Design review of the part shown in the three views and the two pictorial views. Dimensions are in mm from the part's minimum x, y and z. Give positions to 0.01 mm unless a question says otherwise; leave off trailing zeros. Loops run counter-clockwise (first coordinate to the right, second up) from the corner with the lowest first, then second, coordinate; pieces in that order, holes last. Notation, with made-up numbers: (31.25, 44) - (88.25, 44) arc R34 cw to (88.25, 76) - close; hole circle Ø7 at (-12, 36.25). An arc over 180 degrees is marked (long way). Answer in a Markdown table with one row per item.
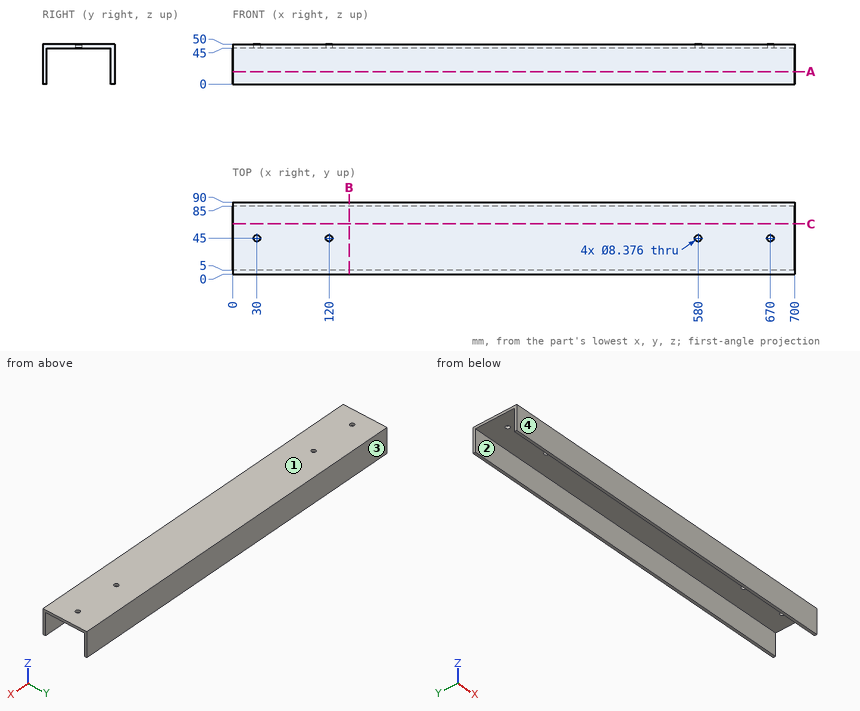
1. Wall thickness on line 1 (X direction, y = 45, z = 48.3); line 2 (Y direction, x = 563.5, z = 15.5); line 3 (Z direction, x = 207, y = 60.5): over which ranges is each line inside the solid? List them lowest first. Write a range as [from, to].
Values:
| item | result |
|---|---|
| line 1 | x = [0, 25.81], [34.19, 115.81], [124.19, 575.81], [584.19, 665.81], [674.19, 700] |
| line 2 | y = [0, 5], [85, 90] |
| line 3 | z = [45, 50] |
2. Clearance check with flat-ended pins moving along their axes: pin 1 (9.5 mm diameter, centred on x = 30, y = 45, fed in from +Z); pin 2 (1.5 mm diameter, centred on x = 471.5, y = 80.5, fed in from -Z). State where each tip first meets the part, or that it passes through.
Values:
| item | result |
|---|---|
| pin 1 | stops at z = 50 |
| pin 2 | stops at z = 45 |
3. We need section C-C, the plane y = 63. Give the boundary of the cut face in (x, z), and give its area (3 significant figures).
Values:
| item | result |
|---|---|
| outline | (0, 45) - (700, 45) - (700, 50) - (0, 50) - close |
| area | 3,500 mm^2 |
4. We need section A-A, the plane z = 15.5. Give the boundary of the cut face in (x, y), and give its area (3 significant figures).
Values:
| item | result |
|---|---|
| outline | (0, 0) - (700, 0) - (700, 5) - (0, 5) - close; (0, 85) - (700, 85) - (700, 90) - (0, 90) - close |
| area | 7,000 mm^2 |
5. Mouldability with a two-part tool opening along Y and no side actions: class the marked faces 1, 2, 3 and 4 as released by +Y, released by -Y, zero draft, split by the parting line, or undercut.
Values:
| item | result |
|---|---|
| face 1 | zero draft |
| face 2 | undercut |
| face 3 | released by +Y |
| face 4 | released by -Y |
6. We need section B-B, the plane x = 145. Give the boundary of the cut face in (y, z), and give its area (3 significant figures).
Values:
| item | result |
|---|---|
| outline | (0, 0) - (5, 0) - (5, 45) - (85, 45) - (85, 0) - (90, 0) - (90, 50) - (0, 50) - close |
| area | 900 mm^2 |
